Autodesk Inventor part; units mm, degrees
ref_plane "YZ Plane" through (0, 0, 0) normal (1, 0, 0) x (0, 1, 0)
ref_plane "XZ Plane" through (0, 0, 0) normal (0, 1, 0) x (-1, 0, 0)
ref_plane "XY Plane" through (0, 0, 0) normal (0, 0, 1) x (1, 0, 0)
sketch "Sketch1" plane through (0, 0, 0) normal (0, 0, 1) x (1, 0, 0)
  line L0 (0, 0) -> (0, -12.7) construction
  line L1 (0, -12.7) -> (0, -31.75) construction
  line L2 (0, 6.35) -> (0, 0) construction
  line L3 (-50.8, -19.05) -> (152.4, -19.05) construction
  line L4 (82.169, 0) -> (183.769, 0) construction
  line L5 (183.769, 0) -> (183.769, -38.1) construction
  line L6 (183.769, -38.1) -> (82.169, -38.1) construction
  line L7 (82.169, -38.1) -> (82.169, 0) construction
  line L8 (183.769, 0) -> (183.769, -38.1)
  line L9 (183.769, -38.1) -> (82.169, -38.1)
  line L10 (79.1709, -6.35) -> (0, -6.35) construction
  line L11 (0, -6.35) -> (0, -12.7)
  line L12 (0, -12.7) -> (82.169, -38.1)
  line L13 (0, -6.35) -> (79.1709, -6.35)
  line L14 (97.8671, 0) -> (183.769, 0)
  line L15 (84.8505, -5.0092) -> (92.1875, -1.3408)
  arc A0 (79.1709, -6.35) -> (84.8505, -5.0092) centre (79.1709, 6.35) ccw
  arc A1 (97.8671, 0) -> (92.1875, -1.3408) centre (97.8671, -12.7) ccw
  point P0 (120.269, -19.05)
  point P1 (145.669, -19.05)
  point P2 (171.069, -19.05)
  dimension "d25" = 12.7
  dimension "d26" = 19.05
  dimension "d27" = 82.169
  dimension "d30" = 203.2
  dimension "d32" = 152.4
  dimension "d34" = 101.6
  dimension "d35" = 38.1
  dimension "d36" = 38.1
  dimension "d37" = 25.4
  dimension "d38" = 25.4
  dimension "d39" = 12.7
  dimension "d98" = 6.35
  dimension "d100" = 12.7
  dimension "d101" = 63.435
  dimension "d102" = 72.823
  dimension "d103" = 38.1
  dimension "d104" = 6.35
  dimension "d105" = 79.1709
extrude "Extrusion1" add sketch "Sketch1" against normal blind 12.7
hole "Hole7" at (120.269, -19.05, 0) at (145.669, -19.05, 0) at (171.069, -19.05, 0) direction (0, 0, -1) diameter 6.5278 end through all
properties part number "Y_shaft_support_brace" material "Aluminum 6061"
For this review, take the finished solid that the model builds, in its own axes (mm). Round coordinates to 2 decimals unless told otherwise and drop trailing zeros. Write each loop counter-clockwise with the first axis right and the second up, starting at its lowest first coordinate (ties: lowest second). Pieces come first, ordered by that corner, then holes. Notation, with made-up numbers: (62.5, 32) - (84.5, 32) arc R24 ccw to (84.5, 46) - close; hole circle Ø1 at (33, 70). An arc over 180 degrees is marked (long way). Answer as a JSON object with one key per item and string values.
1. We need section B-B on y = -19.05. Give the boundary of the cut face in (x, z), then the cut area to 3 significant figures.
Response values:
{"outline": "(20.54, -12.7) - (117.01, -12.7) - (117.01, 0) - (20.54, 0) - close; (123.53, -12.7) - (142.41, -12.7) - (142.41, 0) - (123.53, 0) - close; (148.93, -12.7) - (167.81, -12.7) - (167.81, 0) - (148.93, 0) - close; (174.33, -12.7) - (183.77, -12.7) - (183.77, 0) - (174.33, 0) - close", "area": "1,820 mm2"}
2. We need section D-D on x = 19.5. Give the boundary of the cut face in (y, z), then the cut area to 3 significant figures.
Response values:
{"outline": "(-18.73, -12.7) - (-6.35, -12.7) - (-6.35, 0) - (-18.73, 0) - close", "area": "157 mm2"}
3. For pin 1 Ø6 at (x, y) = (120.269, -19.05) entering from +Z; pin 2 Ø5 at (x, z) = (70.5, -1.5) entering from +Y, all flat-tipped, find the tip position at first contact; note any pin that passes through.
Response values:
{"pin 1": "passes through", "pin 2": "stops at y = -6.35"}
4. We need section C-C on y = -33. Give the boundary of the cut face in (x, z), then the cut area to 3 significant figures.
Response values:
{"outline": "(65.67, -12.7) - (183.77, -12.7) - (183.77, 0) - (65.67, 0) - close", "area": "1,500 mm2"}
5. To check wall thickness, follow line 1 along X through (y, z) = (-5, -5.25); line 2 along Y through (x, z) = (15.5, -10); line 3 along Y through (x, z) = (29.5, -8.5). State the ranges of each line that lie inside material, in increasing order.
Response values:
{"line 1": "x = 84.87 to 183.77", "line 2": "y = -17.49 to -6.35", "line 3": "y = -21.82 to -6.35"}
6. We need section A-A on z = -8.25. Give the boundary of the cut face in (x, y).
Response values:
{"outline": "(0, -12.7) - (82.17, -38.1) - (183.77, -38.1) - (183.77, 0) - (97.87, 0) arc R12.7 ccw to (92.19, -1.34) - (84.85, -5.01) arc R12.7 cw to (79.17, -6.35) - (0, -6.35) - close; hole circle Ø6.53 at (120.27, -19.05); hole circle Ø6.53 at (145.67, -19.05); hole circle Ø6.53 at (171.07, -19.05)"}
7. Draft analysis for pull direction Y (two halves, no side actions). For faces 1 (the face through (148.565, -20.556, -6.439)), 2 (the face through (111, -19, -12.7)), 3 (the face through (39, -6.35, -6)), state which applies: +Y half, -Y half, draft (parallel to the pull), parting line (faces both ways), or undercut.
Response values:
{"face 1": "undercut", "face 2": "draft", "face 3": "+Y half"}
